from build123d import *

# Parameters (mm, degrees)
BOSS_EXTRUDE2_DEPTH = 47
SKETCH2_R           = 4.5
CUT_EXTRUDE1_DEPTH  = 48
CUT_EXTRUDE2_DEPTH  = 6
SKETCH4_R           = 1
CUT_EXTRUDE3_DEPTH  = 6
CUT_EXTRUDE4_DEPTH  = 35
CUT_EXTRUDE5_DEPTH  = 6
BOSS_EXTRUDE3_DEPTH = 0.2
BOSS_EXTRUDE4_DEPTH = 2
SKETCH11_W          = 3.045387933
SKETCH11_H          = 5
CUT_EXTRUDE6_DEPTH  = 35.0000001
FILLET1_R           = 3
FILLET2_R           = 3


with BuildPart() as part:
    # Sketch1 → Boss-Extrude2 (new body)
    with BuildSketch(Plane(origin=(0, 0, 0), x_dir=(1, 0, 0), z_dir=(0, 1, 0))):
        with BuildLine():
            Line((0, 15), (0, 17))
            Line((0, 17), (15, 17))
            ThreePointArc((15, 17), (64, 5.483501156), (113, 17))
            ThreePointArc((113, 17), (162, 5.483501156), (211, 17))
            Line((211, 17), (226, 17))
            Line((226, 17), (226, 15))
            ThreePointArc((226, 15), (211, 0), (226, -15))
            Line((226, -15), (226, -17))
            Line((226, -17), (211, -17))
            ThreePointArc((211, -17), (162, -5.483501156), (113, -17))
            ThreePointArc((113, -17), (64, -5.483501156), (15, -17))
            Line((15, -17), (0, -17))
            Line((0, -17), (0, -15))
            ThreePointArc((0, -15), (15, 0), (0, 15))
        make_face()
    extrude(amount=BOSS_EXTRUDE2_DEPTH)

    # Sketch2 → Cut-Extrude1 (cut, through all)
    with BuildSketch(Plane(origin=(0, 47, 0), x_dir=(1, 0, 0), z_dir=(0, 1, 0))):
        with Locations((113, 0)):
            Circle(SKETCH2_R)
    extrude(amount=-CUT_EXTRUDE1_DEPTH, mode=Mode.SUBTRACT)

    # Sketch3 → Cut-Extrude2 (cut)
    with BuildSketch(Plane(origin=(0, 47, 0), x_dir=(1, 0, 0), z_dir=(0, 1, 0))):
        Polygon((113, -7.794228634), (119.75, -3.897114317), (119.75, 3.897114317), (113, 7.794228634), (106.25, 3.897114317), (106.25, -3.897114317), align=None)
    extrude(amount=-CUT_EXTRUDE2_DEPTH, mode=Mode.SUBTRACT)

    # Sketch4 → Cut-Extrude3 (cut)
    with BuildSketch(Plane(origin=(0, 47, 0), x_dir=(1, 0, 0), z_dir=(0, 1, 0))):
        with Locations((104.25, 0)):
            Circle(SKETCH4_R)
        with Locations((121.75, 0)):
            Circle(SKETCH4_R)
    extrude(amount=-CUT_EXTRUDE3_DEPTH, mode=Mode.SUBTRACT)

    # Sketch5 → Cut-Extrude4 (cut, through all)
    with BuildSketch(Plane(origin=(0, 0, -17), x_dir=(-1, 0, 0), z_dir=(0, 0, -1))):
        with BuildLine():
            Line((-200.749560542, 47), (-128.153486501, 47))
            ThreePointArc((-128.153486501, 47), (-164.451523522, 31.359045891), (-200.749560542, 47))
        make_face()
        with BuildLine():
            ThreePointArc((-25.250439458, 47), (-61.548476478, 31.359045891), (-97.846513499, 47))
            Line((-97.846513499, 47), (-25.250439458, 47))
        make_face()
    extrude(amount=-CUT_EXTRUDE4_DEPTH, mode=Mode.SUBTRACT)

    # Sketch6 → Cut-Extrude5 (cut)
    with BuildSketch(Plane.XZ):
        Polygon((120.505553499, 0), (116.75277675, 6.5), (109.24722325, 6.5), (105.494446501, 0), (109.24722325, -6.5), (116.75277675, -6.5), align=None)
    extrude(amount=-CUT_EXTRUDE5_DEPTH, mode=Mode.SUBTRACT)

    # Sketch7 → Boss-Extrude3 (add)
    with BuildSketch(Plane.XZ.offset(-6)):
        Polygon((120.505553499, 0), (116.75277675, 6.5), (109.24722325, 6.5), (105.494446501, 0), (109.24722325, -6.5), (116.75277675, -6.5), align=None)
    extrude(amount=BOSS_EXTRUDE3_DEPTH)

    # Sketch10 → Boss-Extrude4 (add)
    with BuildSketch(Plane.XZ):
        with BuildLine():
            ThreePointArc((226, -13), (213, 0), (226, 13))
            Line((226, 13), (226, 15))
            ThreePointArc((226, 15), (211, 0), (226, -15))
            Line((226, -15), (226, -13))
        make_face()
    extrude(amount=-BOSS_EXTRUDE4_DEPTH)

    # Sketch11 → Cut-Extrude6 (cut, through all)
    with BuildSketch(Plane(origin=(0, 0, -17), x_dir=(-1, 0, 0), z_dir=(0, 0, -1))):
        with Locations((-19.522693967, 41.5)):
            Rectangle(SKETCH11_W, SKETCH11_H)
        with Locations((-19.522693967, 5.5)):
            Rectangle(SKETCH11_W, SKETCH11_H)
        with Locations((-206.477306033, 5.5)):
            Rectangle(SKETCH11_W, SKETCH11_H)
        with Locations((-206.477306033, 41.5)):
            Rectangle(SKETCH11_W, SKETCH11_H)
    extrude(amount=-CUT_EXTRUDE6_DEPTH, mode=Mode.SUBTRACT)

    # Fillet1
    fillet1_edges = [part.edges().sort_by_distance(p)[0] for p in [
        (18, 41.5, -15.563533182),
        (18, 5.5, -15.563533182),
    ]]
    fillet(fillet1_edges, radius=FILLET1_R)

    # Fillet2
    fillet2_edges = [part.edges().sort_by_distance(p)[0] for p in [
        (18, 41.5, 15.563533182),
        (18, 5.5, 15.563533182),
        (208, 5.5, -15.563533182),
        (208, 5.5, 15.563533182),
        (208, 41.5, -15.563533182),
        (208, 41.5, 15.563533182),
    ]]
    fillet(fillet2_edges, radius=FILLET2_R)


solid = part.part
Model file for the job. Use its own axes, mm. A direction names the side the tool comes from. Give positions to 0.01 mm unless a question says otherwise; leave off trailing zeros. Order: outer loops, then holes, each group sorted by start corner. A loop starts at its lowest first (then second) coordinate and runs counter-clockwise, first axis right, second up. Notation, with made-up numbers: (63.5, 15.5) - (79.5, 15.5) arc R34 cw to (79.5, 50.5) - close; hole circle Ø10 at (58, -15.5). An arc over 180 degrees is marked (long way). Return JSON: item names as keys, results as strings.
1) Pull direction Z, two halves, no side cores. Call faces 5 (the flat face through (18, 5, 0)), 6 (the flat face through (106.25, 44, 0)), 7 (the cylindrical face through (161.289, 17.949, -5.486)): pulls with the +Z half, pulls with the -Z half, needs draft (parallel to the pull), parting line crosses it, or undercut.
Geometry says:
{"face 5": "needs draft", "face 6": "undercut", "face 7": "pulls with the -Z half"}
2) Probe line 1 (Y direction, x = 206, z = 7); line 2 (Z direction, x = 104, y = 45); line 3 (Z direction, x = 113, y = 19). List the from-to ranges inside material, lowest first. Write a range as from..to.
Geometry says:
{"line 1": "0..3, 8..39, 44..47", "line 2": "-13.01..-0.97, 0.97..13.01", "line 3": "-17..-4.5, 4.5..17"}
3) Cut at A-A, the plane y = 16.5. Give the cut face in (x, z), plus the area to 3 significant figures.
Geometry says:
{"outline": "(0, -17) - (15, -17) arc R110 cw to (113, -17) arc R110 cw to (211, -17) - (226, -17) - (226, -15) arc R15 cw to (226, 15) - (226, 17) - (211, 17) arc R110 cw to (113, 17) arc R110 cw to (15, 17) - (0, 17) - (0, 15) arc R15 cw to (0, -15) - close; hole circle Ø9 at (113, 0)", "area": "3,870 mm²"}
4) Flat gauge pins, fed straight in: P1, Ø7, axis at x = 112, z = -1.5, coming from the +Y side; P2, Ø2.5, axis at x = 207.5, z = -4, coming from the -Y side; P3, Ø4, axis at x = 85.5, y = 24.5, coming from the -Z side; P4, Ø12, axis at x = 151.5, z = -9.5, coming from the +Y side. Where does each tip first touch, or does it go through?
Geometry says:
{"P1": "y = 41", "P2": "y = 0", "P3": "z = -8.02", "P4": "y = 34.8"}
5) Cut at C-C, the plane x = 164. Give the cut face in (y, z), plus the area to 3 significant figures.
Geometry says:
{"outline": "(0, -5.5) - (31.36, -5.5) - (31.36, 5.5) - (0, 5.5) - close", "area": "345 mm²"}
6) 3-axis set-ups, long thin cutter, end or side, ignore diameter. For faces 1 (the flat face through (119.75, 44, 0)), 2 (the flat face through (16, 47, 0)), 3 (the flat face through (21.045, 41, 0)), 4 (the flat face through (118.6, 2.9, -3.3)): which of +Z, -Z, +X, -X, +Y, -Y reach the whole face in a straight line?
Geometry says:
{"face 1": "+Y", "face 2": "+Z, -Z, +X, -X, +Y", "face 3": "+Z, -Z", "face 4": "-Y"}
7) Cut at B-B, the plane x = 138.5. Give the cut face in (y, z), plus the area to 3 significant figures.
Geometry says:
{"outline": "(0, -8.02) - (38.63, -8.02) - (38.63, 8.02) - (0, 8.02) - close", "area": "620 mm²"}
